Could you check a few things on this model? Use its own coordinates, in mm. Give positions to 0.01 mm unless a question says otherwise; leave off trailing zeros. Loops run counter-clockwise (first coordinate to the right, second up) from the corner with the lowest first, then second, coordinate; pieces in that order, holes last. Notation, with made-up numbers: (-40, -18) -> (-12, -18) arc R10 cw to (-12, -7) -> close; hole circle Ø6 at (83, 32.5). An arc over 180 degrees is marked (long way). Put each result on its own line as item: value.
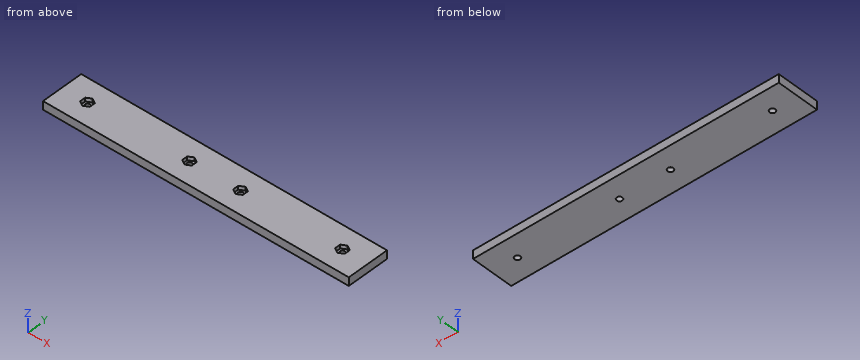
```python
from build123d import *

# Parameters (mm, degrees)
SKETCH1_W           = 179.9
SKETCH1_H           = 24.9
SKETCH1_R           = 1.65
BOSS_EXTRUDE1_DEPTH = 4.9
CUT_EXTRUDE1_DEPTH  = 2.2


with BuildPart() as part:
    # Sketch1 → Boss-Extrude1 (new body)
    with BuildSketch(Plane.XY):
        with Locations((130.907132516, 5.230027325)):
            Rectangle(SKETCH1_W, SKETCH1_H)
        with Locations((205.907132516, 5.230027325)):
            Circle(SKETCH1_R, mode=Mode.SUBTRACT)
        with Locations((145.907132516, 5.230027325)):
            Circle(SKETCH1_R, mode=Mode.SUBTRACT)
        with Locations((115.907132516, 5.230027325)):
            Circle(SKETCH1_R, mode=Mode.SUBTRACT)
        with Locations((55.907132516, 5.230027325)):
            Circle(SKETCH1_R, mode=Mode.SUBTRACT)
    extrude(amount=BOSS_EXTRUDE1_DEPTH)

    # Sketch2 → Cut-Extrude1 (cut)
    with BuildSketch(Plane.XY.offset(4.9)):
        Polygon((58.757132516, 3.584579057), (58.757132516, 6.875475592), (55.907132516, 8.520923859), (53.057132516, 6.875475592), (53.057132516, 3.584579057), (55.907132516, 1.93913079), align=None)
        Polygon((118.757132516, 3.584579057), (118.757132516, 6.875475592), (115.907132516, 8.520923859), (113.057132516, 6.875475592), (113.057132516, 3.584579057), (115.907132516, 1.93913079), align=None)
        Polygon((148.757132516, 3.584579057), (148.757132516, 6.875475592), (145.907132516, 8.520923859), (143.057132516, 6.875475592), (143.057132516, 3.584579057), (145.907132516, 1.93913079), align=None)
        Polygon((208.757132516, 3.584579057), (208.757132516, 6.875475592), (205.907132516, 8.520923859), (203.057132516, 6.875475592), (203.057132516, 3.584579057), (205.907132516, 1.93913079), align=None)
    extrude(amount=-CUT_EXTRUDE1_DEPTH, mode=Mode.SUBTRACT)


solid = part.part
```
1. I need wall thicknesses on line 1 (X direction, y = 5.5, z = 2.15); line 2 (X direction, y = 7.25, z = 3.5); line 3 (Y direction, x = 115, z = 1.8). Which ranges of each line are inside material? Lowest first, please.
Recorded:
line 1: x = 40.96 to 54.28, 57.53 to 114.28, 117.53 to 144.28, 147.53 to 204.28, 207.53 to 220.86
line 2: x = 40.96 to 53.71, 58.11 to 113.71, 118.11 to 143.71, 148.11 to 203.71, 208.11 to 220.86
line 3: y = -7.22 to 3.85, 6.61 to 17.68
2. If we section it at A-A (z = 4.05): List the corners of the cut face in (x, y) for me.
Recorded:
outline: (40.96, -7.22) -> (220.86, -7.22) -> (220.86, 17.68) -> (40.96, 17.68) -> close; hole (53.06, 3.58) -> (55.91, 1.94) -> (58.76, 3.58) -> (58.76, 6.88) -> (55.91, 8.52) -> (53.06, 6.88) -> close; hole (113.06, 3.58) -> (115.91, 1.94) -> (118.76, 3.58) -> (118.76, 6.88) -> (115.91, 8.52) -> (113.06, 6.88) -> close; hole (143.06, 3.58) -> (145.91, 1.94) -> (148.76, 3.58) -> (148.76, 6.88) -> (145.91, 8.52) -> (143.06, 6.88) -> close; hole (203.06, 3.58) -> (205.91, 1.94) -> (208.76, 3.58) -> (208.76, 6.88) -> (205.91, 8.52) -> (203.06, 6.88) -> close
3. I'm going to push flat-ended pins straight in: pin 1 (4.5 mm diameter, centred on x = 116, y = 6, fed in from +Z); pin 2 (3 mm diameter, centred on x = 205.91, y = 5.23, fed in from +Z); pin 3 (1.7 mm diameter, centred on x = 206, y = 6.5, fed in from +Z). Where does each tip first touch, or does it pass through?
Recorded:
pin 1: stops at z = 4.9
pin 2: passes through
pin 3: stops at z = 2.7
